from build123d import *

# Parameters (mm, degrees)
F2_DEPTH = 12.7
F1_R     = 20.5223839117
F3_DEPTH = 12.7
F4_COUNT = 8
F7_DEPTH = 12.7
F6_R     = 43.0741036452
F8_DEPTH = 12.7
F9_COUNT = 15


with BuildPart() as f2:
    # F0 (on Front) → F2 (new body)
    with BuildSketch(Plane.XZ):
        with BuildLine():
            Line((-5.8162368315, 19.3805601989), (6.8837631685, 19.3805601989))
            ThreePointArc((6.8837631685, 19.3805601989), (5.6466426807, 24.8479538456), (2.1762996585, 29.250178249))
            Line((2.1762996585, 29.250178249), (-1.1087733216, 29.250178249))
            ThreePointArc((-1.1087733216, 29.250178249), (-4.5791163438, 24.8479538456), (-5.8162368315, 19.3805601989))
        make_face()
    extrude(amount=F2_DEPTH)

    # F1 (on Front) → F3 (join)
    with BuildSketch(Plane.XZ):
        Circle(F1_R)
    extrude(amount=F3_DEPTH)

    # F4: F2 ×8 about axis
    f4_axis = Axis((0, 0, 0), (0, 1, 0))


with BuildPart() as f2_1:
    add(f2.part)
    for i in range(1, F4_COUNT):
        add(f2.part.rotate(f4_axis, i * 360 / F4_COUNT))


with BuildPart() as f7:
    # F5 (on Front) → F7 (new body)
    with BuildSketch(Plane.XZ):
        with BuildLine():
            Line((-96.6539090335, 40.7748068149), (-83.9539090335, 40.7748068149))
            ThreePointArc((-83.9539090335, 40.7748068149), (-85.1910295213, 46.2422004616), (-88.6613725435, 50.644424865))
            Line((-88.6613725435, 50.644424865), (-91.9464455236, 50.644424865))
            ThreePointArc((-91.9464455236, 50.644424865), (-95.4167885458, 46.2422004616), (-96.6539090335, 40.7748068149))
        make_face()
    extrude(amount=F7_DEPTH)

    # F6 (on Front) → F8 (join)
    with BuildSketch(Plane.XZ):
        with Locations((-88.5588899255, 0)):
            Circle(F6_R)
    extrude(amount=F8_DEPTH)

    # F9: F7 ×15 about axis
    f9_axis = Axis((-88.5588899255, 0, 0), (0, 1, 0))


with BuildPart() as f7_1:
    add(f7.part)
    for i in range(1, F9_COUNT):
        add(f7.part.rotate(f9_axis, i * 360 / F9_COUNT))


solid = f2_1.part
Geometry check sheet. Reference: the model listing, model coordinates, mm. A direction names the side the tool comes from. Coordinates: 2 decimals unless noted, no trailing zeros. Order: outer loops, then holes, each group sorted by start corner. A loop starts at its lowest first (then second) coordinate and runs counter-clockwise, first axis right, second up. Notation, with made-up numbers: (44, 42) -> (67, 42) arc R7 cw to (67, 55) -> close; hole circle Ø6 at (57, -24). An arc over 180 degrees is marked (long way). Use a Markdown table: item, result. Add a question column.
1. Cross-section at B-B (x = -15). Enter the section's corners in (y, z).
2. Set-up check for faces 5 (the face through (25.05, -6.26, 4.48)), 6 (the face through (-21.077, -6.261, -20.289)), 7 (the face through (0, 0, 0)), 8 (the face through (-5.68, -6.26, -24.78)), 9 (the face through (5.68, -6.26, 24.78)): record each of +Z, -Z, +X, -X, +Y, -Y from which the full face is reachable in a straight line by a thin tool's end or side.
3. Material ranges on L1, parallel to Z at x = -20, y = -4.25; L2, parallel to X at y = -3.25, z = -24; L3, parallel to Z at x = 17, y = -3.5, recorded low to high.
4. Mould release check, pull along Z, two halves, no side actions. Record for faces 1 (the face through (-25.05, -6.26, -4.48)), 2 (the face through (20.289, -6.261, -21.077)), 3 (the face through (21.536, -6.261, 13.503)), 4 (the face through (14.548, -6.261, 20.882)): pulls with the +Z half, pulls with the -Z half, needs draft (parallel to the pull), parting line crosses it, or undercut.
5. Go/stop test with flat-tipped pins: pin 1 Ø8 at (x, z) = (-1.5, 6.5) entering from +Y; pin 2 Ø5 at (x, y) = (-23, -11) entering from +Z; pin 3 Ø4 at (x, y) = (-12.5, -9.5) entering from -Z; pin 4 Ø2 at (x, y) = (-6.5, -11) entering from -Z. Record where each tip stops, or that it passes through.
6. Cross-section at A-A (z = 11). Enter the section's corners in (x, y).
Filled sheet:
| question | item | result |
|---|---|---|
| 1 | outline | (-12.7, -21.02) -> (0, -21.02) -> (0, 21.98) -> (-12.7, 21.98) -> close |
| 2 | face 5 | +X, +Y, -Y |
| 2 | face 6 | -Z, -X, +Y, -Y |
| 2 | face 7 | +Z, -Z, +X, -X, +Y |
| 2 | face 8 | -Z, +Y, -Y |
| 2 | face 9 | +Z, +Y, -Y |
| 3 | L1 | -21.37 to -10.54, -5.8 to 6.87, 12.52 to 21.37 |
| 3 | L2 | -6.01 to 4.95 |
| 3 | L3 | -22.27 to 21.44 |
| 4 | face 1 | undercut |
| 4 | face 2 | pulls with the -Z half |
| 4 | face 3 | undercut |
| 4 | face 4 | pulls with the +Z half |
| 5 | pin 1 | y = 0 |
| 5 | pin 2 | z = 20.87 |
| 5 | pin 3 | z = -20.87 |
| 5 | pin 4 | z = -25.15 |
| 6 | outline | (-19.03, -12.7) -> (20.31, -12.7) -> (20.31, 0) -> (-19.03, 0) -> close |
